from build123d import *

# Parameters (mm, degrees)
SKETCH1_W           = 7
SKETCH1_H           = 79
SKETCH1_R           = 2
BOSS_EXTRUDE1_DEPTH = 3
SKETCH2_W           = 7
SKETCH2_H           = 3
BOSS_EXTRUDE2_DEPTH = 7
CUT_EXTRUDE1_REACH  = 81.707
BOSS_EXTRUDE3_DEPTH = 1


with BuildPart() as part:
    # Sketch1 → Boss-Extrude1 (new body)
    with BuildSketch(Plane.XY):
        Rectangle(SKETCH1_W, SKETCH1_H)
        with Locations((0, -30.5)):
            Circle(SKETCH1_R, mode=Mode.SUBTRACT)
        with Locations((0, 33.5)):
            Circle(SKETCH1_R, mode=Mode.SUBTRACT)
    extrude(amount=BOSS_EXTRUDE1_DEPTH)

    # Sketch2 → Boss-Extrude2 (add)
    with BuildSketch(Plane.XY.offset(3)):
        with Locations((0, -38)):
            Rectangle(SKETCH2_W, SKETCH2_H)
    extrude(amount=BOSS_EXTRUDE2_DEPTH)

    # Sketch3 → Cut-Extrude1 (cut, up to next)
    with BuildSketch(Plane.XZ.offset(39.5), mode=Mode.PRIVATE) as cut_extrude1_sk1:
        with BuildLine():
            Line((-2, 6.5), (-2, 10))
            Line((-2, 10), (2, 10))
            Line((2, 10), (2, 6.5))
            ThreePointArc((2, 6.5), (0, 4.5), (-2, 6.5))
        make_face()
    cut_extrude1_tool1 = extrude(cut_extrude1_sk1.sketch, amount=-CUT_EXTRUDE1_REACH, mode=Mode.PRIVATE) & part.part
    add(cut_extrude1_tool1.solids().sort_by_distance((0, -39.5, 7.444953))[0], mode=Mode.SUBTRACT)

    # Sketch4 → Boss-Extrude3 (add)
    with BuildSketch(Plane.ZY.offset(3.5)):
        Polygon((3, -33.839487464), (5.660512536, -36.5), (3, -36.5), align=None)
    boss_extrude3 = extrude(amount=-BOSS_EXTRUDE3_DEPTH)

    # Mirror1: Boss-Extrude3 across plane
    add(boss_extrude3.mirror(Plane.ZY))


solid = part.part
Can you work these out from the model? Positions are in its coordinate system, mm. A direction names the side the tool comes from. Give positions to 0.01 mm unless a question says otherwise; leave off trailing zeros. Loops run counter-clockwise (first coordinate to the right, second up) from the corner with the lowest first, then second, coordinate; pieces in that order, holes last. Notation, with made-up numbers: (74.25, 38) -> (89.25, 38) arc R13 cw to (89.25, 61) -> close; hole circle Ø1 at (38.25, 74). An arc over 180 degrees is marked (long way). Return JSON: item names as keys, results as strings.
Q1. I want a section at D-D, the plane y = 24. List the corners of the cut face in (x, z) for me, then the cut area to 3 significant figures.
Checks:
{"outline": "(-3.5, 0) -> (3.5, 0) -> (3.5, 3) -> (-3.5, 3) -> close", "area": "21.0 mm2"}
Q2. I need wall thicknesses on probe 1 along Y at (x, z) = (0, 1); probe 2 along Y at (x, z) = (-0.75, 1.25); probe 3 along Z at (x, y) = (-2.25, -9.5). Which ranges of each line are inside material? Lowest first, please.
Checks:
{"probe 1": "y = -39.5 to -32.5, -28.5 to 31.5, 35.5 to 39.5", "probe 2": "y = -39.5 to -32.35, -28.65 to 31.65, 35.35 to 39.5", "probe 3": "z = 0 to 3"}
Q3. On a 3-axis mill with a long thin cutter (end or side, diameter ignored), from which of +Z, -Z, +X, -X, +Y, -Y can I reach the whole of each face in a straight line? I mean faces 4 (the face through (2.5, -36, 4)), 5 (the face through (3, -38, 10)), 6 (the face through (2, -38, 8)). Say none if no direction works.
Checks:
{"face 4": "+Z, +Y", "face 5": "+Z, +X, -X, +Y, -Y", "face 6": "+Z, +Y, -Y"}
Q4. I want a section at B-B, the plane y = 33.5. List the corners of the cut face in (x, z) for me, then the cut area to 3 significant figures.
Checks:
{"outline": "(-3.5, 0) -> (-2, 0) -> (-2, 3) -> (-3.5, 3) -> close; (2, 0) -> (3.5, 0) -> (3.5, 3) -> (2, 3) -> close", "area": "9.00 mm2"}
Q5. We'd pull the mould along X, two halves only. Please class faces 1 (the face through (-3, -38, 10)), 2 (the face through (-3.5, -3, 2)), 3 (the face through (-2, -38, 8)): released by +X, released by -X, zero draft, split by the parting line, or undercut.
Checks:
{"face 1": "zero draft", "face 2": "released by -X", "face 3": "undercut"}
Q6. For pin 1 Ø3 at (y, z) = (-35, 5) entering from +X; pin 2 Ø2 at (x, y) = (-1, 7.5) entering from +Z, each with a flat end and sliding along its axis, tell me the tip position at first contact or that it passes through.
Checks:
{"pin 1": "stops at x = 3.5", "pin 2": "stops at z = 3"}
Q7. I want a section at C-C, the plane z = 1. List the corners of the cut face in (x, y) for me, then the cut area to 3 significant figures.
Checks:
{"outline": "(-3.5, -39.5) -> (3.5, -39.5) -> (3.5, 39.5) -> (-3.5, 39.5) -> close; hole circle Ø4 at (0, -30.5); hole circle Ø4 at (0, 33.5)", "area": "528 mm2"}
Q8. I want a section at A-A, the plane x = 0. List the corners of the cut face in (y, z) for me.
Checks:
{"outline": "(-39.5, 0) -> (-32.5, 0) -> (-32.5, 3) -> (-36.5, 3) -> (-36.5, 4.5) -> (-39.5, 4.5) -> close; (-28.5, 0) -> (31.5, 0) -> (31.5, 3) -> (-28.5, 3) -> close; (35.5, 0) -> (39.5, 0) -> (39.5, 3) -> (35.5, 3) -> close"}
